For this review, take the finished solid that the model builds, in its own axes (mm). A direction names the side the tool comes from. Round coordinates to 2 decimals unless told otherwise and drop trailing zeros. Order: outer loops, then holes, each group sorted by start corner. A loop starts at its lowest first (then second) coordinate and runs counter-clockwise, first axis right, second up.
Autodesk Inventor part; units mm, degrees
ref_plane "YZ Plane" through (0, 0, 0) normal (1, 0, 0) x (0, 1, 0)
ref_plane "XZ Plane" through (0, 0, 0) normal (0, 1, 0) x (-1, 0, 0)
ref_plane "XY Plane" through (0, 0, 0) normal (0, 0, 1) x (1, 0, 0)
sketch "Sketch1" plane through (0, 0, 0) normal (0, 0, 1) x (1, 0, 0)
  line L0 (-27, 25) -> (27, 25)
  line L1 (27, 25) -> (27, -25)
  line L2 (27, -25) -> (-27, -25)
  line L3 (-27, -25) -> (-27, 25)
  point P0 (0, 0)
  dimension "d0" = 54
  dimension "d1" = 50
  dimension "d2" = 25
  dimension "d3" = 27
extrude "Base" add sketch "Sketch1" along normal blind 4
sketch "Sketch2" plane through (0, 0, 4) normal (0, 0, 1) x (1, 0, 0)
  line L0 (-27, -25) -> (-27, 25)
  line L1 (0, 23.0221) -> (0, -15.4934) construction
  line L2 (-23.6958, 0) -> (15.7708, 0) construction
  line L3 (-27, 7.5) -> (-23, 7.5)
  line L4 (-23, 7.5) -> (-23, -7.5)
  line L5 (-23, -7.5) -> (-27, -7.5)
  line L6 (-27, -7.5) -> (-27, 7.5)
  line L7 (-27, 25) -> (-23, 25)
  line L8 (-23, 25) -> (-23, 22.5)
  line L9 (-23, 22.5) -> (-27, 22.5)
  line L10 (-27, 22.5) -> (-27, 25)
  line L11 (-27, -25) -> (-23, -25)
  line L12 (-23, -25) -> (-23, -22.5)
  line L13 (-23, -22.5) -> (-27, -22.5)
  line L14 (-27, -22.5) -> (-27, -25)
  line L15 (27, 7.5) -> (23, 7.5)
  line L16 (23, 7.5) -> (23, -7.5)
  line L17 (23, -7.5) -> (27, -7.5)
  line L18 (27, -7.5) -> (27, 7.5)
  line L19 (27, 25) -> (23, 25)
  line L20 (23, 25) -> (23, 22.5)
  line L21 (23, 22.5) -> (27, 22.5)
  line L22 (27, 22.5) -> (27, 25)
  line L23 (27, -25) -> (23, -25)
  line L24 (23, -25) -> (23, -22.5)
  line L25 (23, -22.5) -> (27, -22.5)
  line L26 (27, -22.5) -> (27, -25)
  point P0 (0, 0)
  point P1 (23.6958, 0)
  dimension "d9" = 4
  dimension "d10" = 15
  dimension "d11" = 4
  dimension "d13" = 7.5
  dimension "d14" = 15
  dimension "d15" = 15
  dimension "d16" = 4
extrude "Sleeves" cut sketch "Sketch2" against normal blind 4
sketch "Sketch3" plane through (0, 0, 4) normal (0, 0, 1) x (1, 0, 0)
  line L0 (0, 0) -> (-5.6569, 5.6569) construction
  line L1 (0, 0) -> (8, 0) construction
  line L2 (0, 0) -> (6.7175, 6.7175) construction
  line L3 (0, 0) -> (-6.7175, -6.7175) construction
  line L4 (0, 0) -> (5.6569, -5.6569) construction
  dimension "d19" = 8
  dimension "d20" = 135
  dimension "d21" = 9.5
  dimension "d22" = 9.5
  dimension "d23" = 8
hole "MotorMounts" at (6.7175, 6.7175, 4) at (-5.6569, 5.6569, 4) at (-6.7175, -6.7175, 4) at (5.6569, -5.6569, 4) direction (0, 0, -1) diameter 3 end through all
sketch "Sketch4" plane through (0, 0, 4) normal (0, 0, 1) x (1, 0, 0)
  circle A0 centre (0, 0) radius 4.5
  dimension "d31" = 9
extrude "ShaftClearance" cut sketch "Sketch4" against normal through all
sketch "Sketch5" plane through (0, 0, 4) normal (0, 0, 1) x (1, 0, 0)
  circle A0 centre (0, 0) radius 4.5
  line L0 (-23, 7.5) -> (-23, -7.5)
  line L1 (23, -7.5) -> (23, 7.5)
  line L2 (-23, 1.5) -> (-18, 1.5)
  line L3 (-18, 1.5) -> (-18, 3.5)
  line L4 (-18, 3.5) -> (-15, 3.5)
  line L5 (-15, 3.5) -> (-15, 1.5)
  line L6 (-15, 1.5) -> (-13, 1.5)
  line L7 (-13, 1.5) -> (-13, -1)
  line L8 (-13, -1) -> (-15, -1)
  line L9 (-15, -1) -> (-15, -3)
  line L10 (-15, -3) -> (-18, -3)
  line L11 (-18, -3) -> (-18, -1.4035)
  line L12 (-18, -1.4035) -> (-23, -1.4035)
  line L13 (-23, -1.4035) -> (-23, 1.5)
  dimension "d34" = 5
  dimension "d35" = 2
  dimension "d36" = 3
  dimension "d37" = 2
  dimension "d38" = 2.5
  dimension "d39" = 2
  dimension "d40" = 3
  dimension "d41" = 1.5
extrude "ScrewLock" cut sketch "Sketch5" against normal blind 10 contours L2 L3 L4 L5 L6 L7 L8 L9 L10 L11 L12 L0
mirror "ScrewLockDoubler" about plane through (0, 0, 0) normal (1, 0, 0) of "ScrewLock"
sketch "Sketch6" plane through (0, 0, 4) normal (0, 0, 1) x (1, 0, 0)
  line L0 (-23, 25) -> (23, 25)
  line L1 (-23, 25) -> (-23, 22.5)
  line L2 (18, 3.5) -> (18, 1.5)
  line L3 (-18, 20) -> (-6, 20)
  line L4 (-6, 20) -> (-6, 15)
  line L5 (-18, 20) -> (-18, 8)
  line L6 (15, 3.5) -> (18, 3.5)
  circle A0 centre (0, 0) radius 4.5
  arc A1 (-6, 15) -> (-14.0357, 8) centre (0, 0) ccw
  line L7 (-14.0357, 8) -> (-18, 8)
  dimension "d44" = 5
  dimension "d45" = 12
  dimension "d46" = 12
  dimension "d48" = 5
  dimension "d49" = 5
extrude "CornerCutout" cut sketch "Sketch6" against normal blind 10 contours L3 L4 A1 L7 L5
sketch "Sketch7" plane through (0, 0, 4) normal (0, 0, 1) x (1, 0, 0)
  line L0 (-18, 8) -> (-18, 20)
  line L1 (-18, 20) -> (-6, 20)
  arc A0 (-6, 15) -> (-14.0357, 8) centre (0, 0) ccw
  line L2 (18, 3.5) -> (18, 1.5)
  circle A1 centre (0, 0) radius 4.5
  line L3 (0, 0) -> (-18.1317, 23.2182) construction
  line L4 (0, 0) -> (-21.2105, 20.4919) construction
  line L5 (0, 0) -> (-18, 20) construction
  line L6 (-15.6185, 20) -> (-9.9435, 12.7329)
  line L7 (-15.6185, 20) -> (-18, 20)
  line L8 (-18, 17.3902) -> (-18, 20)
  line L9 (-18, 17.3902) -> (-11.6188, 11.2251)
  arc A2 (-9.9435, 12.7329) -> (-11.6188, 11.2251) centre (0, 0) ccw
  dimension "d52" = 8
  dimension "d54" = 4
extrude "DiagonalSupport" add sketch "Sketch7" against normal blind 4 contours L0 L1 L6 A0 L9
mirror "CornerDoubler" about plane through (0, 0, 0) normal (0, 1, 0) of "CornerCutout", "DiagonalSupport"
mirror "CornerQuadrupler" about plane through (0, 0, 0) normal (1, 0, 0) of "CornerCutout", "CornerDoubler", "DiagonalSupport"
properties part number "MotorSupport"
(1) Tool access review of faces 1 (the face through (-25, 7.5, 2)), 2 (the face through (13, 0, 2)), 3 (the face through (-14.854, 14.351, 2.028)): name each direction out of +Z, -Z, +X, -X, +Y, -Y from which nothing blocks a thin tool from reaching the whole face with its end or side.
(2) Add section B-B on x = 0. Give the boundary of the cut face in (y, z).
(3) Draft analysis for pull direction X (two halves, no side actions). For faces 4 (the face through (25, 7.5, 2)), 5 (the face through (12.945, 9.666, 2.028)), 6 (the face through (18, -2, 2)), 7 (the face through (23, 5, 2)), state which applies: pulls with the +X half, pulls with the -X half, needs draft (parallel to the pull), parting line crosses it, or undercut.
(4) Wall thickness on L1, parallel to Y at x = 0, z = 2.25; L2, parallel to X at y = -17, z = 3.8; L3, parallel to Y at x = 7, z = 3.1: over which ranges is each line inside the solid? List them lowest first.
(5) Add section D-D on z = 1.15. Count the separate pieces of the cut face and the enclosed holes in it, plus the area to 3 significant figures.
(6) Add section C-C on x = -17. Give the boundary of the cut face in (y, z), plus the area to 3 significant figures.
(7) Add section A-A on y = 0. Give the boundary of the cut face in (x, z).
(8) Clearance check with flat-ended pins moving along their axes: P1, Ø1.2, axis at y = 24, z = 1, coming from the -X side; P2, Ø2, axis at x = -25.5, z = 1.5, coming from the +Y side; P3, Ø1.2, axis at x = -25.5, z = 2.5, coming from the -Y side. State where each tip first meets the part, or that it passes through.
Here are the results:
1. face 1: +Z, -Z, -X
1. face 2: +Z, -Z, +X
1. face 3: +Z, -Z
2. outline: (-25, 0) - (-4.5, 0) - (-4.5, 4) - (-25, 4) - close; (4.5, 0) - (25, 0) - (25, 4) - (4.5, 4) - close
3. face 4: needs draft
3. face 5: undercut
3. face 6: undercut
3. face 7: pulls with the +X half
4. L1: y = -25 to -4.5, 4.5 to 25
4. L2: x = -27 to -18, -17.6 to -13.28, -6 to 6, 13.28 to 17.6, 18 to 27
4. L3: y = -25 to -20, -14.56 to -6.32, -4.99 to 5.24, 8.19 to 14.56, 20 to 25
5. separate pieces: 1
5. enclosed holes: 13
5. area: 2,050 mm2
6. outline: (-25, 0) - (-16.42, 0) - (-16.42, 4) - (-25, 4) - close; (-8, 0) - (-3, 0) - (-3, 4) - (-8, 4) - close; (3.5, 0) - (8, 0) - (8, 4) - (3.5, 4) - close; (16.42, 0) - (25, 0) - (25, 4) - (16.42, 4) - close
6. area: 107 mm2
7. outline: (-13, 0) - (-4.5, 0) - (-4.5, 4) - (-13, 4) - close; (4.5, 0) - (13, 0) - (13, 4) - (4.5, 4) - close
8. P1: stops at x = -23
8. P2: stops at y = 22.5
8. P3: stops at y = -22.5
